The drawing under review shows one solid part. Ordinate dimensions are in mm from its lowest x, y, z. A direction names the side the tool comes from. Round coordinates to 2 decimals unless told otherwise and drop trailing zeros. Write each loop counter-clockwise with the first axis right and the second up, starting at its lowest first coordinate (ties: lowest second). Pieces come first, ordered by that corner, then holes. Notation, with made-up numbers: (-7, 3) -> (35, 3) arc R11 cw to (35, 24) -> close; hole circle Ø10 at (64.25, -20.5). An arc over 180 degrees is marked (long way). Use CSV: the item, a comma, the result in double quotes. Start each with the question number.
1) Take a section at C-C, the plane x = 5. Give the boundary of the cut face in (y, z).
2) Mouldability with a two-part tool opening along Y and no side actions: class the marked faces 4, 5 and 6 as released by +Y, released by -Y, zero draft, split by the parting line, or undercut.
3) For pin 1 Ø8 at (x, y) = (21, 37) entering from -Z; pin 2 Ø7 at (x, y) = (37, 21) entering from -Z; pin 3 Ø2 at (x, y) = (36.5, 21) entering from -Z; pin 4 Ø10 at (y, z) = (11, 7) entering from -X, all flat-tipped, find the tip position at first contact; note any pin that passes through.
4) Take a section at A-A, the plane y = 21. Give the boundary of the cut face in (x, z), then the cut area to 3 significant figures.
5) Wall thickness on probe 1 along X at (y, z) = (21, 21); probe 2 along Z at (x, y) = (11, 11.5); probe 3 along Y at (x, z) = (26, 25): over which ranges is each line inside the solid? List them lowest first. Write a range as [from, to].
6) Machinability: for the marked faces 1, 2 and 3, which of the approach directions +Z, -Z, +X, -X, +Y, -Y give a long, thin tool a straight path to every point of the face, cutting with its end or side? Answer none if there is none.
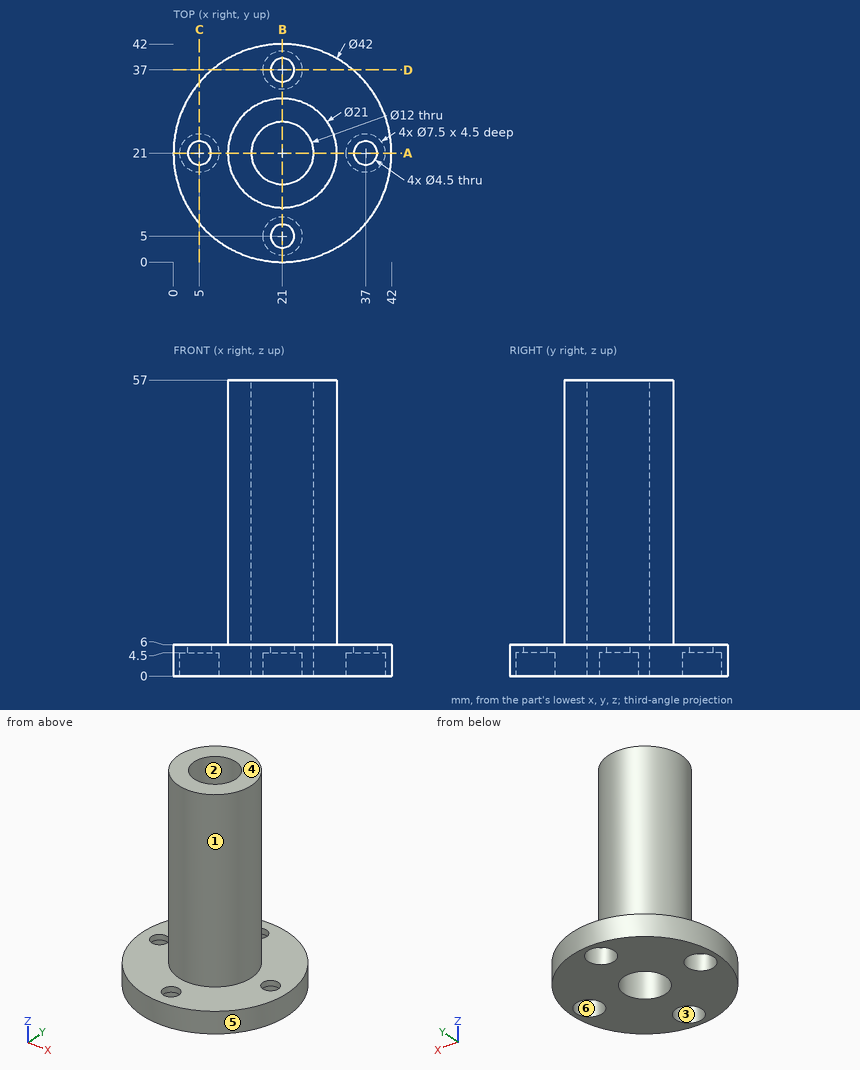
Values found:
1,outline,"(7.4, 0) -> (17.25, 0) -> (17.25, 4.5) -> (18.75, 4.5) -> (18.75, 6) -> (7.4, 6) -> close; (23.25, 4.5) -> (24.75, 4.5) -> (24.75, 0) -> (34.6, 0) -> (34.6, 6) -> (23.25, 6) -> close"
2,face 4,"zero draft"
2,face 5,"split by the parting line"
2,face 6,"undercut"
3,pin 1,"z = 0"
3,pin 2,"z = 4.5"
3,pin 3,"through"
3,pin 4,"x = 0.63"
4,outline,"(0, 0) -> (1.25, 0) -> (1.25, 4.5) -> (2.75, 4.5) -> (2.75, 6) -> (0, 6) -> close; (7.25, 4.5) -> (8.75, 4.5) -> (8.75, 0) -> (15, 0) -> (15, 57) -> (10.5, 57) -> (10.5, 6) -> (7.25, 6) -> close; (27, 0) -> (33.25, 0) -> (33.25, 4.5) -> (34.75, 4.5) -> (34.75, 6) -> (31.5, 6) -> (31.5, 57) -> (27, 57) -> close; (39.25, 4.5) -> (40.75, 4.5) -> (40.75, 0) -> (42, 0) -> (42, 6) -> (39.25, 6) -> close"
4,area,"558 mm²"
5,probe 1,"[10.5, 15], [27, 31.5]"
5,probe 2,"[0, 6]"
5,probe 3,"[11.77, 17.68], [24.32, 30.23]"
6,face 1,"+Z"
6,face 2,"+Z, -Z"
6,face 3,"-Z"
